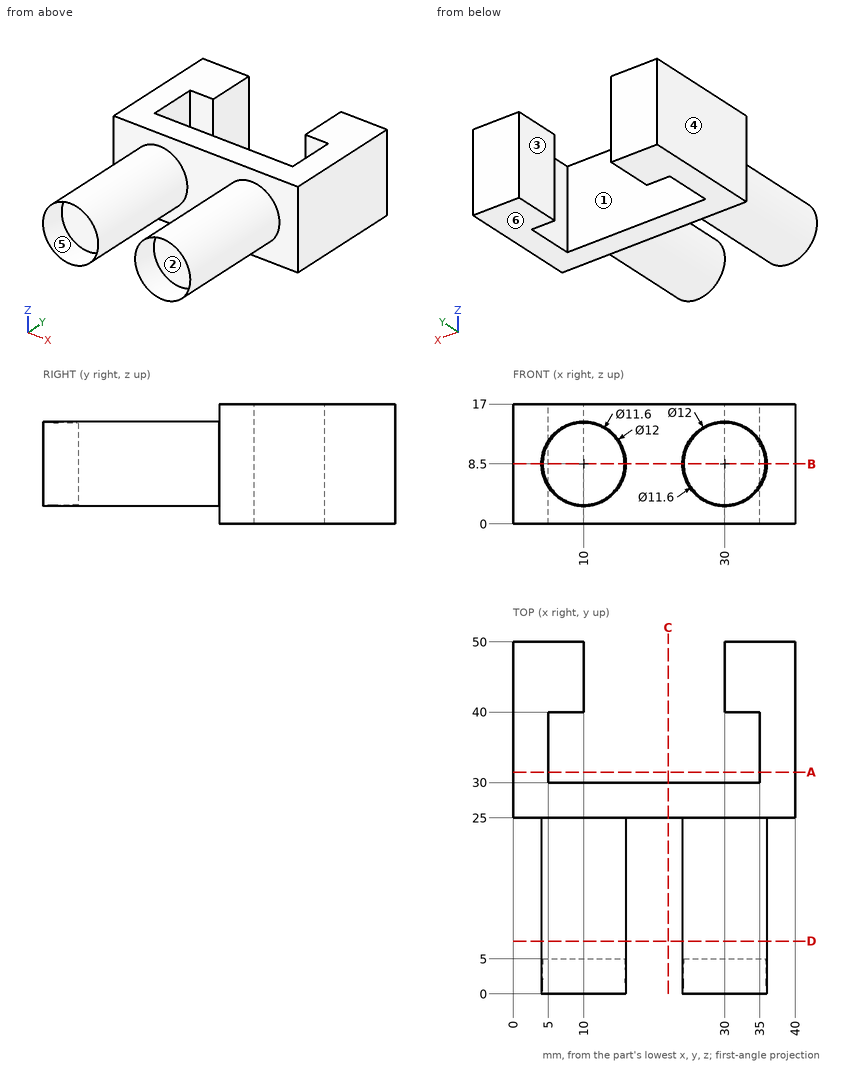
The figure shows three views and two pictorial views of one solid part (mm, origin at its lowest corner). Answer the questions. A direction names the side the tool comes from. Coordinates: 2 decimals unless noted, no trailing zeros. Loops run counter-clockwise (first coordinate to the right, second up) from the corner with the lowest first, then second, coordinate; pieces in that order, holes last.
1) Find section A-A on y = 31.5. Write down the section's boundary in (x, z).
2) Flat-ended cylindrical pins translate along their axes: pin 1 Ø4 at (x, z) = (35.5, 15) entering from -Y; pin 2 Ø1.5 at (x, z) = (8.5, 5) entering from -Y. Find the tip coordinate at first contact, or state that the pin passes through.
3) Find the intervals of material crossed by L1, parallel to Y at x = 8.5, z = 5.75; L2, parallel to X at y = 42, z = 6.5; L3, parallel to X at y = 2.5, z = 13.5, in increasing order.
4) Find section C-C on x = 22. Write down the section's boundary in (y, z).
5) Determine the mould class of the marked faces 4, 5 and 6 for opening direction X: pulls with the +X half, pulls with the -X half, needs draft (parallel to the pull), parting line crosses it, or undercut.
6) Find section D-D on y = 7.5. Write down the section's boundary in (x, z), then the cut area to 3 significant figures.
7) A tool of negligible diameter and unlimited length cuts with its end or side. For the marked faces 1, 2 and 3, from which of +Z, -Z, +X, -X, +Y, -Y can it reach the whole face along a straight path? Write none if from no direction.
8) Find section B-B on z = 8.5. Write down the section's boundary in (x, y).
Values:
1. outline: (0, 0) - (5, 0) - (5, 17) - (0, 17) - close; (35, 0) - (40, 0) - (40, 17) - (35, 17) - close
2. pin 1: stops at y = 25
2. pin 2: stops at y = 5
3. L1: y = 5 to 30, 40 to 50
3. L2: x = 0 to 10, 30 to 40
3. L3: x = 6.68 to 6.87, 13.13 to 13.32, 26.68 to 26.87, 33.13 to 33.32
4. outline: (25, 0) - (30, 0) - (30, 17) - (25, 17) - close
5. face 4: pulls with the -X half
5. face 5: undercut
5. face 6: needs draft
6. outline: circle Ø12 at (10, 8.5); circle Ø12 at (30, 8.5)
6. area: 226 mm2
7. face 1: +Z, -Z
7. face 2: -Y
7. face 3: +Z, -Z, +Y
8. outline: (0, 25) - (4, 25) - (4, 0) - (4.2, 5) - (15.8, 5) - (16, 0) - (16, 25) - (24, 25) - (24, 0) - (24.2, 5) - (35.8, 5) - (36, 0) - (36, 25) - (40, 25) - (40, 50) - (30, 50) - (30, 40) - (35, 40) - (35, 30) - (5, 30) - (5, 40) - (10, 40) - (10, 50) - (0, 50) - close
